Here's how the part is built. I have some questions about the finished solid (model axes, mm). A direction names the side the tool comes from. Coordinates: 2 decimals unless noted, no trailing zeros. Write each loop counter-clockwise with the first axis right and the second up, starting at its lowest first coordinate (ties: lowest second). Pieces come first, ordered by that corner, then holes. Notation, with made-up numbers: M 79,34 L 98,34 A36 ccw 98,69 Z; hole C 78,44 d2. An arc over 180 degrees is marked long. Use a Markdown table: item, result.
```python
from build123d import *

# Parameters (mm, degrees)
F0_R     = 2
F0_R_2   = 1.6
F1_DEPTH = 3


# Not quite as in the source:
# - a feature names something its author has since deleted; it is built from what else it names


with BuildPart() as f1:
    # F0 (on Front) → F1 (new body)
    with BuildSketch(Plane.XZ):
        with BuildLine():
            ThreePointArc((1.7860619516, 39.4986839248), (1.1086440911, 38.8081032796), (0.5768869335, 38))
            Line((0.5768869335, 38), (47.4231130665, 38))
            ThreePointArc((47.4231130665, 38), (46.8913559089, 38.8081032796), (46.2139380484, 39.4986839248))
            Line((46.2139380484, 39.4986839248), (39.8600581363, 44.8302222156))
            ThreePointArc((39.8600581363, 44.8302222156), (38.3562208045, 45.6984631039), (36.6461200879, 46))
            Line((36.6461200879, 46), (11.3538799121, 46))
            ThreePointArc((11.3538799121, 46), (9.6437791955, 45.6984631039), (8.1399418637, 44.8302222156))
            Line((8.1399418637, 44.8302222156), (1.7860619516, 39.4986839248))
        make_face()
        with BuildLine():
            Line((47.4231130665, 38), (0.5768869335, 38))
            ThreePointArc((0.5768869335, 38), (0.1463639747, 36.869385243), (0, 35.6684617092))
            Line((0, 35.6684617092), (0, 5))
            ThreePointArc((0, 5), (1.4644660941, 1.4644660941), (5, 0))
            Line((5, 0), (6.5, 0))
            ThreePointArc((6.5, 0), (10.0355339059, -1.4644660941), (11.5, -5))
            Line((11.5, -5), (11.5, -5.0126606831))
            Line((11.5, -5.0126606831), (11.5, -13.75))
            Line((11.5, -13.75), (36.5, -13.75))
            Line((36.5, -13.75), (36.5, -5))
            ThreePointArc((36.5, -5), (37.9644660941, -1.4644660941), (41.5, 0))
            Line((41.5, 0), (43, 0))
            ThreePointArc((43, 0), (46.5355339059, 1.4644660941), (48, 5))
            Line((48, 5), (48, 35.6684617092))
            ThreePointArc((48, 35.6684617092), (47.8536360253, 36.869385243), (47.4231130665, 38))
        make_face()
        with Locations((9.5, 5.25)):
            Circle(F0_R, mode=Mode.SUBTRACT)
        with Locations((38.5, 5.25)):
            Circle(F0_R, mode=Mode.SUBTRACT)
        with Locations((9.5, 32.75)):
            Circle(F0_R, mode=Mode.SUBTRACT)
        with Locations((24, 35.75)):
            Circle(F0_R_2, mode=Mode.SUBTRACT)
        with Locations((38.5, 32.75)):
            Circle(F0_R, mode=Mode.SUBTRACT)
    extrude(amount=F1_DEPTH)


solid = f1.part
```
1. I need wall thicknesses on probe 1 along X at (y, z) = (-2.05, 6); probe 2 along Z at (x, y) = (38.5, -1.65); probe 3 along X at (y, z) = (-2.4, 34.5). Which ranges of each line are inside material? Lowest first, please.
Answers follow:
| item | result |
|---|---|
| probe 1 | x = 0 to 7.65, 11.35 to 36.65, 40.35 to 48 |
| probe 2 | z = -1 to 3.25, 7.25 to 30.75, 34.75 to 45.64 |
| probe 3 | x = 0 to 8.53, 10.47 to 23, 25 to 37.53, 39.47 to 48 |
2. Suppose I cut it at B-B on x = 24. Write out the boundary of the cut face in (y, z).
Answers follow:
| item | result |
|---|---|
| outline | M -3,-13.75 L 0,-13.75 L 0,34.15 L -3,34.15 Z; M -3,37.35 L 0,37.35 L 0,46 L -3,46 Z |
3. Suppose I cut it at D-D on x = 38.5. Write out the boundary of the cut face in (y, z), and give its area (3 significant figures).
Answers follow:
| item | result |
|---|---|
| outline | M -3,-1 L 0,-1 L 0,3.25 L -3,3.25 Z; M -3,7.25 L 0,7.25 L 0,30.75 L -3,30.75 Z; M -3,34.75 L 0,34.75 L 0,45.64 L -3,45.64 Z |
| area | 116 mm2 |
4. Suppose I cut it at C-C on z = 32.75. Write out the boundary of the cut face in (x, y).
Answers follow:
| item | result |
|---|---|
| outline | M 0,-3 L 7.5,-3 L 7.5,0 L 0,0 Z; M 11.5,-3 L 36.5,-3 L 36.5,0 L 11.5,0 Z; M 40.5,-3 L 48,-3 L 48,0 L 40.5,0 Z |
5. Which directions (+Z, -Z, +X, -X, +Y, -Y) give clear straight access to the entire face, cutting with the end or side of a thin tool? Please do faces 4 (the face through (48, -1, 20)), 5 (the face through (36.5, -1, -9)), 6 (the face through (6, -1, 0)).
Answers follow:
| item | result |
|---|---|
| face 4 | +Z, -Z, +X, +Y, -Y |
| face 5 | -Z, +X, +Y, -Y |
| face 6 | -Z, -X, +Y, -Y |
6. We'd pull the mould along X, two halves only. Please class faces 1 (the face through (0, -1, 21)), 2 (the face through (24, -1, -13.75)), 3 (the face through (8.026, -1.479, 6.602)): +X half, -X half, draft (parallel to the pull), parting line (faces both ways), or undercut.
Answers follow:
| item | result |
|---|---|
| face 1 | -X half |
| face 2 | draft |
| face 3 | undercut |
7. Suppose I cut it at A-A on y = -1.3. Write out the boundary of the cut face in (x, z), and give its area (3 significant figures).
Answers follow:
| item | result |
|---|---|
| outline | M 0,5 A5 ccw 5,0 L 6.5,0 A5 cw 11.5,-5 L 11.5,-13.75 L 36.5,-13.75 L 36.5,-5 A5 cw 41.5,0 L 43,0 A5 ccw 48,5 L 48,35.67 A5 ccw 46.21,39.5 L 39.86,44.83 A5 ccw 36.65,46 L 11.35,46 A5 ccw 8.14,44.83 L 1.79,39.5 A5 ccw 0,35.67 Z; hole C 9.5,5.25 d4; hole C 9.5,32.75 d4; hole C 24,35.75 d3.2; hole C 38.5,5.25 d4; hole C 38.5,32.75 d4 |
| area | 2,410 mm2 |
8. Will these pins go through, and if not, where does the flat tip stop? pin 1 Ø0.8 at (x, y) = (42, -1) entering from -Z; pin 2 Ø0.9 at (y, z) = (-2, -9.5) entering from +X.
Answers follow:
| item | result |
|---|---|
| pin 1 | stops at z = 0 |
| pin 2 | stops at x = 36.5 |
